```python
from build123d import *

# Parameters (mm, degrees)
SKETCH1_R           = 4.5
BOSS_EXTRUDE1_DEPTH = 2.5


with BuildPart() as part:
    # Sketch1 → Boss-Extrude1 (new, symmetric)
    with BuildSketch(Plane.XY):
        with BuildLine():
            Line((0, 9.5), (20.41, 9.5))
            Line((20.41, 9.5), (20.41, -9.5))
            Line((20.41, -9.5), (0, -9.5))
            ThreePointArc((0, -9.5), (-9.5, 0), (0, 9.5))
        make_face()
        Circle(SKETCH1_R, mode=Mode.SUBTRACT)
    extrude(amount=BOSS_EXTRUDE1_DEPTH, both=True)


solid = part.part
```
Here's how the part is built. I have some questions about the finished solid (model axes, mm). Coordinates: 2 decimals unless noted, no trailing zeros. Loops run counter-clockwise (first coordinate to the right, second up) from the corner with the lowest first, then second, coordinate; pieces in that order, holes last. Notation, with made-up numbers: (18, 87.25) -> (31, 87.25) arc R24 cw to (31, 109.25) -> close; hole circle Ø5 at (58, -3). An arc over 180 degrees is marked (long way). Return JSON: item names as keys, results as strings.
1) Thinking about a two-plate mould opening in X: for faces 1 (the face through (9, 0, 2.5)), 2 (the face through (20.41, 0, 0)), 3 (the face through (-0.59, 4.46, -0.04)), 4 (the face through (-9.498, -0.209, 0.035)), which applies, +X half, -X half, draft (parallel to the pull), parting line (faces both ways), or undercut?
Results below:
{"face 1": "draft", "face 2": "+X half", "face 3": "undercut", "face 4": "-X half"}
2) If we section it at A-A, the plane y = 0: Write out the boundary of the cut face in (x, z).
Results below:
{"outline": "(-9.5, -2.5) -> (-4.5, -2.5) -> (-4.5, 2.5) -> (-9.5, 2.5) -> close; (4.5, -2.5) -> (20.41, -2.5) -> (20.41, 2.5) -> (4.5, 2.5) -> close"}
3) If we section it at C-C, the plane z = -1.7: Write out the boundary of the cut face in (x, y).
Results below:
{"outline": "(0, -9.5) -> (20.41, -9.5) -> (20.41, 9.5) -> (0, 9.5) arc R9.5 ccw to start; hole circle Ø9 at (0, 0)"}
4) If we section it at B-B, the plane x = 1: Write out the boundary of the cut face in (y, z).
Results below:
{"outline": "(-9.5, -2.5) -> (-4.39, -2.5) -> (-4.39, 2.5) -> (-9.5, 2.5) -> close; (4.39, -2.5) -> (9.5, -2.5) -> (9.5, 2.5) -> (4.39, 2.5) -> close"}
5) I need wall thicknesses on line 1 (Y direction, x = 0, z = -1.4); line 2 (X direction, y = -2.5, z = -1.4); line 3 (X direction, y = -0.5, z = 0). Which ranges of each line are inside material? Lowest first, please. Write a range as from..to.
Results below:
{"line 1": "-9.5..-4.5, 4.5..9.5", "line 2": "-9.17..-3.74, 3.74..20.41", "line 3": "-9.49..-4.47, 4.47..20.41"}
6) If we section it at D-D, the plane y = -7.25: Write out the boundary of the cut face in (x, z).
Results below:
{"outline": "(-6.14, -2.5) -> (20.41, -2.5) -> (20.41, 2.5) -> (-6.14, 2.5) -> close"}
